Source: CAD feature listing. Evaluate the final solid. Frame: model axes, mm. Face numbers are marked on the shaded views. A direction names the side the tool comes from. Coordinates: 2 decimals unless noted, no trailing zeros. Loops run counter-clockwise (first coordinate to the right, second up) from the corner with the lowest first, then second, coordinate; pieces in that order, holes last. Notation, with made-up numbers: (-18, 40.5) - (20, 40.5) arc R12 ccw to (20, 51.5) - close; hole circle Ø2 at (13.25, -38). An arc over 180 degrees is marked (long way). Write item = value, one per line. Start each with the question number.
from build123d import *

# Parameters (mm, degrees)
HEXAGONSOCKET_DEPTH = 2


with BuildPart() as part:
    # Sketch1 → Base (revolve)
    with BuildSketch(Plane.XY):
        Polygon((0, 0), (8, 0), (8, 0.625), (6.125, 2.5), (0.433, 2.5), (0, 2.067), align=None)
    revolve(axis=Axis((-14.774129749, 0, 0), (1, 0, 0)))

    # Sketch2 → HexagonSocket (cut)
    with BuildSketch(Plane(origin=(0, 0.220293087, -0.139195271), x_dir=(0, 0, 1), z_dir=(-1, 0, 0))):
        Polygon((1.582570944, -0.220293087), (0.860883108, 1.029706913), (-0.582492565, 1.029706913), (-1.304180402, -0.220293087), (-0.582492565, -1.470293087), (0.860883108, -1.470293087), align=None)
    extrude(amount=-HEXAGONSOCKET_DEPTH, mode=Mode.SUBTRACT)

    # Sketch3 → Cut-Revolve (revolve, cut)
    with BuildSketch(Plane.XY):
        Polygon((2, 1.25), (2.721687836, 0), (2, 0), align=None)
    revolve(axis=Axis((2, 0, 0), (-1, 0, 0)), mode=Mode.SUBTRACT)


solid = part.part
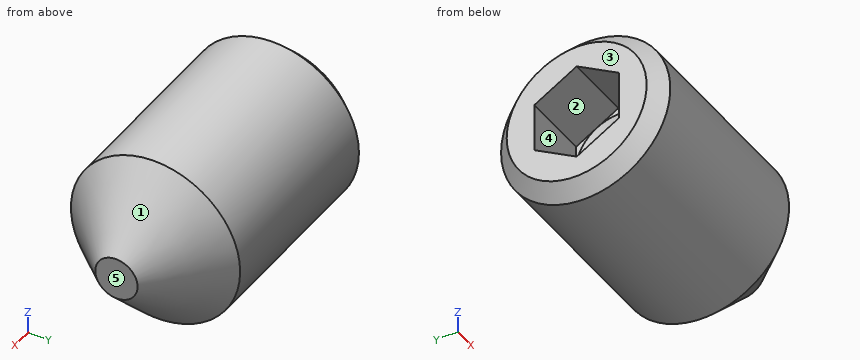
Item 1: Reachability of the marked faces 4 and 5 from +Z, -Z, +X, -X, +Y, -Y: full face, straight path, thin tool, end or side. Return the list, or none.
Item 2: First-contact query: pin 1 (1 mm diameter, centred on y = 1.5, z = 1.5, fed in from -X). Flat tip, straight axial feed; report the tip coordinate or a pass-through.
Item 3: Material intervals for L1, parallel to Y at x = 1.5, z = -0.95; L2, parallel to X at y = 0.45, z = 0.65; L3, parallel to X at y = 0.85, z = -2.1, sorted ascending. Write a range as [from, to].
Item 4: Cut plane B-B (x = 6.5). Return the cut outline in (y, z) (3 decimals).
Item 5: Cut plane A-A (x = 2.5). Return the cut outline in (y, z).
Item 6: Draft query along Z for the marked faces 1, 2 and 3. Return one class per face: released by +Z, released by -Z, zero draft, split by the parting line, or undercut.
Responses:
q1.face_4 = -X
q1.face_5 = +Z, -Z, +X, +Y, -Y
q2.pin_1 = 0
q3.L1 = [-2.31, -0.85], [0.85, 2.31]
q3.L2 = [2.27, 7.83]
q3.L3 = [0.2, 6.36]
q4.outline = circle Ø4.25 at (0, 0)
q5.outline = circle Ø5 at (0, 0); hole circle Ø0.77 at (0, 0)
q6.face_1 = split by the parting line
q6.face_2 = undercut
q6.face_3 = zero draft
